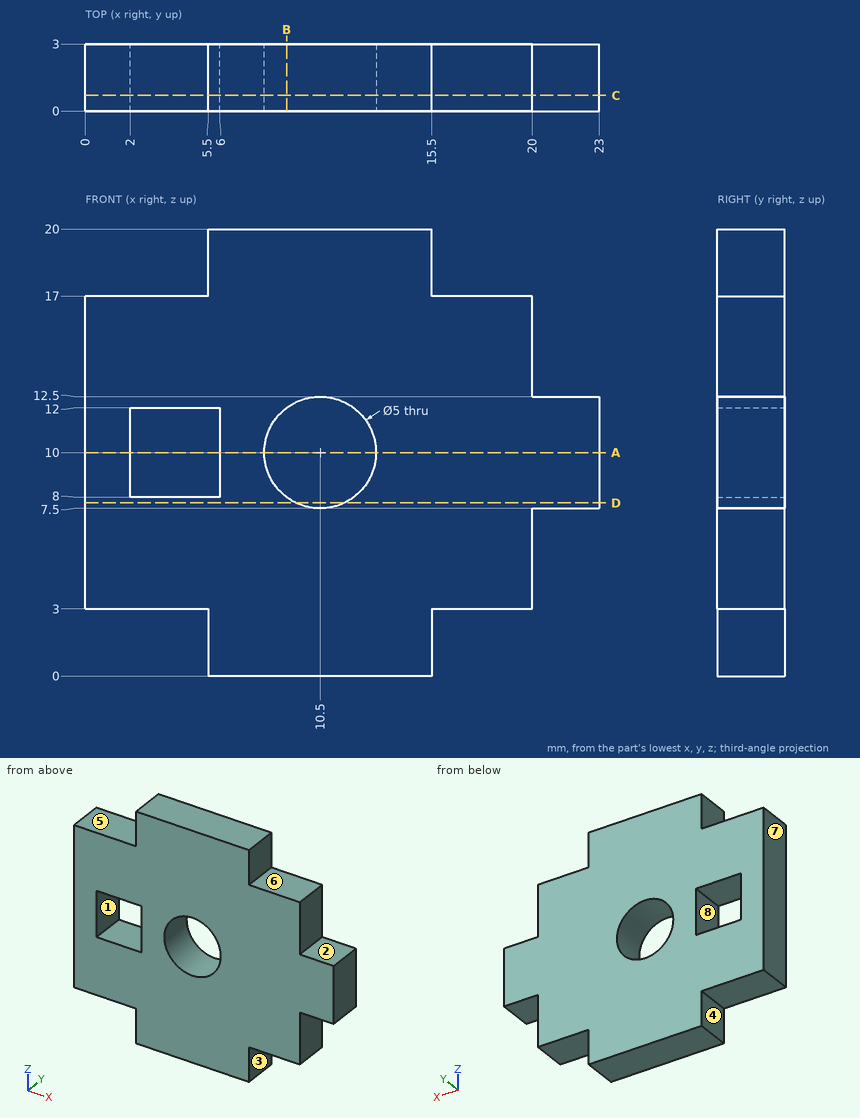
For this review, use the dimensioned drawing (mm, ordinates from the lowest corner) and the shaded views. A direction names the side the tool comes from. Round coordinates to 2 decimals unless told otherwise and drop trailing zeros. Write each loop counter-clockwise with the first axis right and the second up, starting at its lowest first coordinate (ties: lowest second). Pieces come first, ordered by that corner, then holes. Notation, with made-up numbers: M 34,9.25 L 48,9.25 A23 cw 48,26.25 Z; hole C 69,-19.5 d11. An arc over 180 degrees is marked long. Answer as CSV lines item,"result". Start each with the question number.
Q1. The part is to be moulded in two halves that separate along Z. For the marked faces 6, 7 and 8, say which applies: +Z half, -Z half, draft (parallel to the pull), parting line (faces both ways), or undercut.
Q2. Wall thickness on line 1 along Z through (x, y) = (5.25, 1); line 2 along X through (y, z) = (2.3, 9); line 3 along Z through (x, y) = (10.5, 1.65): over which ranges is each line inside the solid? List them lowest first.
Q3. Consider section C-C, the plane y = 0.7. Give the boundary of the cut face in (x, z).
Q4. Tool access review of the marked faces 1, 2, 3, 4 and 5: name each direction out of +Z, -Z, +X, -X, +Y, -Y from which nothing blocks a thin tool from reaching the whole face with its end or side.
Q5. Consider section D-D, the plane z = 7.75. Give the boundary of the cut face in (x, y).
Q6. Clearance check with flat-ended pins moving along their axes: P1, Ø1.5, axis at x = 21.5, y = 2, coming from the -Z side; P2, Ø0.9, axis at y = 1.5, z = 1.5, coming from the -X side; P3, Ø0.9, axis at y = 2, z = 1.5, coming from the +X side; P4, Ø3, axis at x = 10.5, z = 10, coming from the -Y side. State where each tip first meets the part, or that it passes through.
Q7. Consider section B-B, the plane x = 9. Give the boundary of the cut face in (y, z), then the cut area to 3 significant figures.
Q8. Consider section A-A, the plane z = 10. Give the boundary of the cut face in (x, y).
Result set:
1,face 6,"+Z half"
1,face 7,"draft"
1,face 8,"undercut"
2,line 1,"z = 3 to 8, 12 to 17"
2,line 2,"x = 0 to 2, 6 to 8.21, 12.79 to 23"
2,line 3,"z = 0 to 7.5, 12.5 to 20"
3,outline,"M 0,3 L 5.5,3 L 5.5,0 L 15.5,0 L 15.5,3 L 20,3 L 20,7.5 L 23,7.5 L 23,12.5 L 20,12.5 L 20,17 L 15.5,17 L 15.5,20 L 5.5,20 L 5.5,17 L 0,17 Z; hole M 2,8 L 6,8 L 6,12 L 2,12 Z; hole C 10.5,10 d5"
4,face 1,"+Y, -Y"
4,face 2,"+Z, +X, +Y, -Y"
4,face 3,"-Z, +X, +Y, -Y"
4,face 4,"-Z, -X, +Y, -Y"
4,face 5,"+Z, -X, +Y, -Y"
5,outline,"M 0,0 L 9.41,0 L 9.41,3 L 0,3 Z; M 11.59,0 L 23,0 L 23,3 L 11.59,3 Z"
6,P1,"stops at z = 7.5"
6,P2,"stops at x = 5.5"
6,P3,"stops at x = 15.5"
6,P4,"passes through"
7,outline,"M 0,0 L 3,0 L 3,8 L 0,8 Z; M 0,12 L 3,12 L 3,20 L 0,20 Z"
7,area,"48.0 mm²"
8,outline,"M 0,0 L 2,0 L 2,3 L 0,3 Z; M 6,0 L 8,0 L 8,3 L 6,3 Z; M 13,0 L 23,0 L 23,3 L 13,3 Z"
